```python
from build123d import *

# Parameters (mm, degrees)
F0_W     = 40
F0_H     = 40
F1_DEPTH = 3
F2_W     = 12
F2_H     = 6
F3_DEPTH = 3
F5_D     = 2
F5_DEPTH = 10


with BuildPart() as f1:
    # F0 (on Top) → F1 (new body)
    with BuildSketch(Plane.XY):
        Rectangle(F0_W, F0_H)
    extrude(amount=-F1_DEPTH)

    # F2 (on face) → F3 (cut)
    with BuildSketch(Plane(origin=(0, 0, -3), x_dir=(1, 0, 0), z_dir=(0, 0, -1))):
        with Locations((5, 13)):
            Rectangle(F2_W, F2_H)
    extrude(amount=-F3_DEPTH, mode=Mode.SUBTRACT)

    # F5
    with Locations(Plane.XY):
        with Locations((-17, 17), (17, 17), (14, 14), (-14, 14), (-17, -17), (-14, -14), (14, -14), (17, -17)):
            Hole(F5_D / 2, depth=F5_DEPTH)


solid = f1.part
```
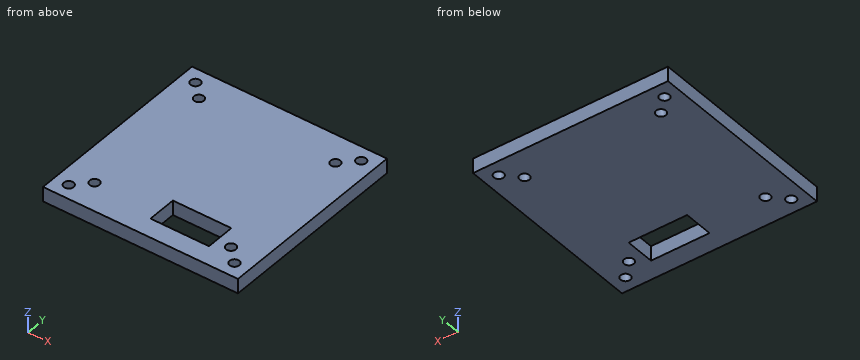
The listing builds one solid part. Answer for the finished solid, in the listing's coordinates (mm). Round coordinates to 2 decimals unless told otherwise and drop trailing zeros. Write each loop counter-clockwise with the first axis right and the second up, starting at its lowest first coordinate (ties: lowest second). Pieces come first, ordered by that corner, then holes. Notation, with made-up numbers: (76.25, 73.25) -> (110.25, 73.25) arc R32 ccw to (110.25, 105.25) -> close; hole circle Ø4 at (60, 64.5). An arc over 180 degrees is marked (long way). Use CSV: the item, a comma, the result in double quotes. Start each with the question number.
(1) Section D-D on z = -1.9 is taken. Count the separate pieces of the cut face and the enclosed holes in it, then the cut area to 3 significant figures.
(2) Section C-C on x = -17 is taken. Give the vertices of the cut face in (y, z).
(3) Consider L1, parallel to Y at x = -17, z = -2; L2, parallel to Y at x = -14, z = -0.65; L3, parallel to X at y = -11.5, z = -2.55. Determine where each line is inside the solid, lowest interval first. Write a range as from..to.
(4) Section B-B on x = 9 is taken. Give the vertices of the cut face in (y, z).
(5) Section A-A on y = -14 is taken. Give the vertices of the cut face in (x, z).
(6) This flat-tipped pin is pushed along its axis until it touches: pin 1 (1.6 mm diameter, centred on x = -17, y = -17, fed in from +Z). Where does it stop, or does it pass through?
A:
1,separate pieces,"1"
1,enclosed holes,"9"
1,area,"1,500 mm²"
2,outline,"(-20, -3) -> (-18, -3) -> (-18, 0) -> (-20, 0) -> close; (-16, -3) -> (16, -3) -> (16, 0) -> (-16, 0) -> close; (18, -3) -> (20, -3) -> (20, 0) -> (18, 0) -> close"
3,L1,"y = -20..-18, -16..16, 18..20"
3,L2,"y = -20..-15, -13..13, 15..20"
3,L3,"x = -20..-1, 11..20"
4,outline,"(-20, -3) -> (-16, -3) -> (-16, 0) -> (-20, 0) -> close; (-10, -3) -> (20, -3) -> (20, 0) -> (-10, 0) -> close"
5,outline,"(-20, -3) -> (-15, -3) -> (-15, 0) -> (-20, 0) -> close; (-13, -3) -> (-1, -3) -> (-1, 0) -> (-13, 0) -> close; (11, -3) -> (13, -3) -> (13, 0) -> (11, 0) -> close; (15, -3) -> (20, -3) -> (20, 0) -> (15, 0) -> close"
6,pin 1,"passes through"
